Job drawing, mm, ordinate dimensions from the low corner. One solid piece. A direction names the side the tool comes from. Round coordinates to 2 decimals unless told otherwise and drop trailing zeros. Order: outer loops, then holes, each group sorted by start corner. A loop starts at its lowest first (then second) coordinate and runs counter-clockwise, first axis right, second up. Notation, with made-up numbers: (87.25, 36) -> (105.25, 36) arc R18 cw to (105.25, 67) -> close; hole circle Ø1 at (66, 6). An arc over 180 degrees is marked (long way). Write item = value, one per line.
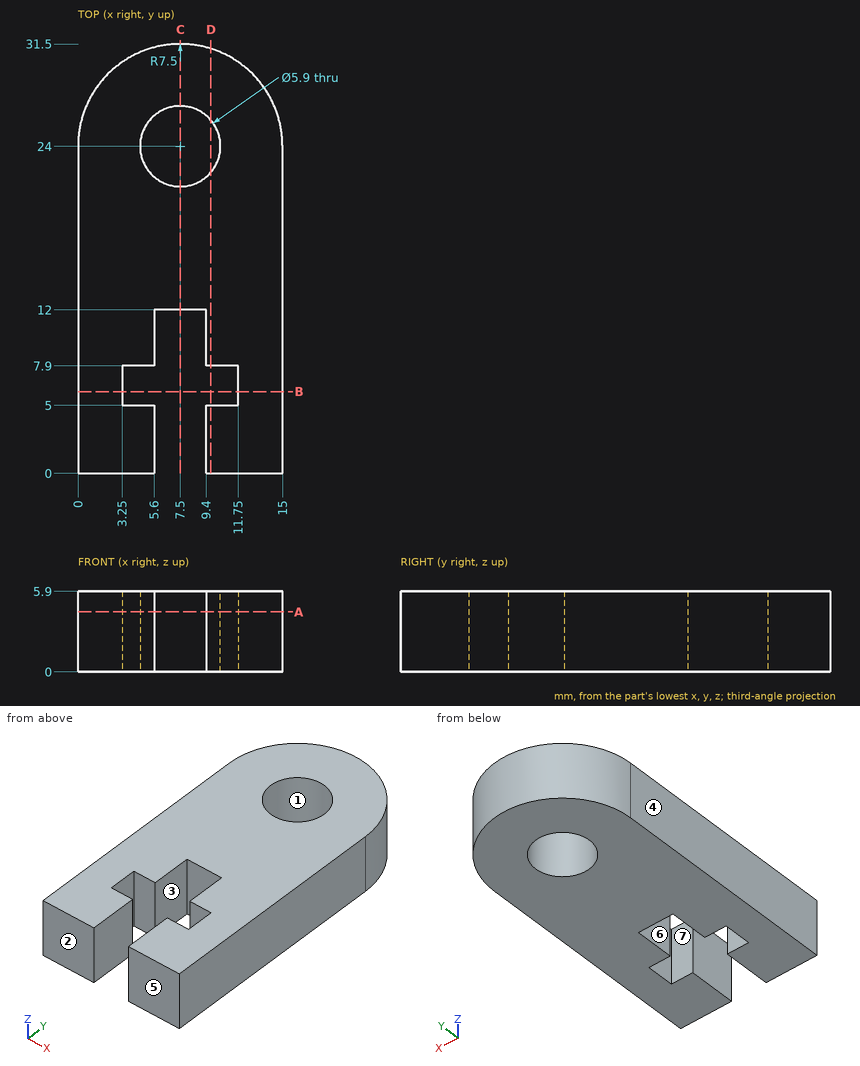
Q1. Cut at A-A, the plane z = 4.4. List the corners of the cut face in (x, y).
Check values:
outline = (0, 0) -> (5.6, 0) -> (5.6, 5) -> (3.25, 5) -> (3.25, 7.9) -> (5.6, 7.9) -> (5.6, 12) -> (9.4, 12) -> (9.4, 7.9) -> (11.75, 7.9) -> (11.75, 5) -> (9.4, 5) -> (9.4, 0) -> (15, 0) -> (15, 24) arc R7.5 ccw to (0, 24) -> close; hole circle Ø5.9 at (7.5, 24)
Q2. Flat gauge pins, fed straight in: pin 1 (1.2 mm diameter, centred on x = 10.5, z = 4, fed in from +Y); pin 2 (1 mm diameter, centred on x = 2.5, z = 4.5, fed in from +Y); pin 3 (1.1 mm diameter, centred on x = 6.5, z = 3, fed in from -Y); pin 4 (5.5 mm diameter, centred on x = 7.5, y = 24, fed in from -Z). Where does each tip first touch, or does it go through?
Check values:
pin_1 = 31.11
pin_2 = 30
pin_3 = 12
pin_4 = through
Q3. Cut at C-C, the plane x = 7.5. List the corners of the cut face in (y, z).
Check values:
outline = (12, 0) -> (21.05, 0) -> (21.05, 5.9) -> (12, 5.9) -> close; (26.95, 0) -> (31.5, 0) -> (31.5, 5.9) -> (26.95, 5.9) -> close
Q4. Mould opens along X. For the marked faces 1, 2, 3 and 4 say: released by +X, released by -X, zero draft, split by the parting line, or undercut.
Check values:
face_1 = undercut
face_2 = zero draft
face_3 = undercut
face_4 = released by -X
Q5. Which spindle directions (+Z, -Z, +X, -X, +Y, -Y) get a long thin tool onto all of the face, cutting with end or side? Do the marked faces 5, 6 and 7. Say none if no direction does.
Check values:
face_5 = +Z, -Z, +X, -X, -Y
face_6 = +Z, -Z, -Y
face_7 = +Z, -Z
Q6. Cut at B-B, the plane y = 6. List the corners of the cut face in (x, z).
Check values:
outline = (0, 0) -> (3.25, 0) -> (3.25, 5.9) -> (0, 5.9) -> close; (11.75, 0) -> (15, 0) -> (15, 5.9) -> (11.75, 5.9) -> close
Q7. Probe probe 1 along Y at (x, z) = (7.5, 4.2); probe 2 along X at (y, z) = (10.5, 3.4); probe 3 along Y at (x, z) = (5, 3.6). List the from-to ranges inside material, lowest first.
Check values:
probe_1 = 12 to 21.05, 26.95 to 31.5
probe_2 = 0 to 5.6, 9.4 to 15
probe_3 = 0 to 5, 7.9 to 22.43, 25.57 to 31.07
Q8. Cut at D-D, the plane x = 9.75. List the corners of the cut face in (y, z), and give its area (3 significant figures).
Check values:
outline = (0, 0) -> (5, 0) -> (5, 5.9) -> (0, 5.9) -> close; (7.9, 0) -> (22.09, 0) -> (22.09, 5.9) -> (7.9, 5.9) -> close; (25.91, 0) -> (31.15, 0) -> (31.15, 5.9) -> (25.91, 5.9) -> close
area = 144 mm²
